from build123d import *

# Parameters (mm, degrees)
F0_R     = 203.2
F0_R_2   = 8.89
F1_DEPTH = 20.32


with BuildPart() as f1:
    # F0 (on Front) → F1 (new body)
    with BuildSketch(Plane.XZ):
        Circle(F0_R)
        with Locations((-134.703841816, -134.703841816)):
            Circle(F0_R_2, mode=Mode.SUBTRACT)
        with Locations((0, -190.5)):
            Circle(F0_R_2, mode=Mode.SUBTRACT)
        with Locations((-190.5, 0)):
            Circle(F0_R_2, mode=Mode.SUBTRACT)
        with Locations((134.703841816, -134.703841816)):
            Circle(F0_R_2, mode=Mode.SUBTRACT)
        with Locations((190.5, 0)):
            Circle(F0_R_2, mode=Mode.SUBTRACT)
        with BuildLine():
            ThreePointArc((-123.8970573285, 144.2619540188), (-120.3869637363, 158.4652267944), (-108.347947169, 150.1516358339))
            ThreePointArc((-108.347947169, 150.1516358339), (-114.0889306017, 141.8380448734), (-123.8970573285, 144.2619540188))
        make_face(mode=Mode.SUBTRACT)
        with Locations((0, 190.5)):
            Circle(F0_R_2, mode=Mode.SUBTRACT)
        with Locations((117.237947169, 150.1516358339)):
            Circle(F0_R_2, mode=Mode.SUBTRACT)
    extrude(amount=F1_DEPTH)


solid = f1.part
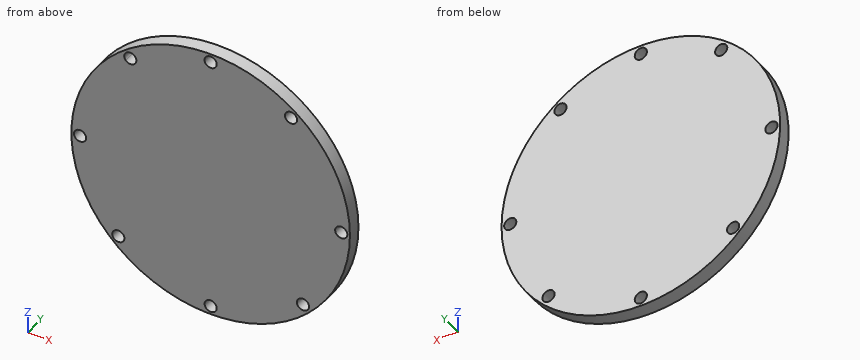
Could you check a few things on this model? Use its own coordinates, in mm. Coordinates: 2 decimals unless noted, no trailing zeros. Order: outer loops, then holes, each group sorted by start corner. A loop starts at its lowest first (then second) coordinate and runs counter-clockwise, first axis right, second up. Notation, with made-up numbers: (66.25, 32.25) - (105.25, 32.25) arc R12 cw to (105.25, 42.25) - close; hole circle Ø4 at (62, -12). An arc over 180 degrees is marked (long way). Answer in a Markdown table with one row per item. Add a question column.
(1) If we section it at A-A, the plane z = 0: Please give me the cut outline in (x, y), then the cut area to 3 significant figures.
(2) If we section it at D-D, the plane z = -190.5: Please give me the cut outline in (x, y), then the cut area to 3 significant figures.
(3) Will these pins go through, and if not, where does the flat tip stop? pin 1 (10.5 mm diameter, centred on x = -190.5, z = 0, fed in from +Y); pin 2 (1.5 mm diameter, centred on y = -15.5, z = -116, fed in from +X); pin 3 (5 mm diameter, centred on y = -16.5, z = 12.5, fed in from -X); pin 4 (1.5 mm diameter, centred on y = -10.5, z = 25, fed in from +X).
(4) If we section it at C-C, the plane y = -10.5: State how many separate pieces and enclosed holes the cut face has, then the cut area to 3 significant figures.
(5) If we section it at B-B, the plane x = 119: Please give me the cut outline in (y, z), then the cut area to 3 significant figures.
(6) I need wall thicknesses on L1, parallel to Z at x = 0, y = -15.75; L2, parallel to X at y = -8.5, z = 148; L3, parallel to Z at x = -127, y = -11.5. Which ranges of each line are inside material? Lowest first, please.
Results are:
| question | item | result |
|---|---|---|
| 1 | outline | (-203.2, -20.32) - (-199.39, -20.32) - (-199.39, 0) - (-203.2, 0) - close; (-181.61, -20.32) - (181.61, -20.32) - (181.61, 0) - (-181.61, 0) - close; (199.39, -20.32) - (203.2, -20.32) - (203.2, 0) - (199.39, 0) - close |
| 1 | area | 7,540 mm2 |
| 2 | outline | (-70.71, -20.32) - (-8.89, -20.32) - (-8.89, 0) - (-70.71, 0) - close; (8.89, -20.32) - (70.71, -20.32) - (70.71, 0) - (8.89, 0) - close |
| 2 | area | 2,510 mm2 |
| 3 | pin 1 | passes through |
| 3 | pin 2 | stops at x = 167.35 |
| 3 | pin 3 | stops at x = -202.95 |
| 3 | pin 4 | stops at x = 201.75 |
| 4 | separate pieces | 1 |
| 4 | enclosed holes | 8 |
| 4 | area | 128,000 mm2 |
| 5 | outline | (-20.32, -164.71) - (0, -164.71) - (0, 141.44) - (-20.32, 141.44) - close; (-20.32, 158.87) - (0, 158.87) - (0, 164.71) - (-20.32, 164.71) - close |
| 5 | area | 6,340 mm2 |
| 6 | L1 | z = -203.2 to -199.39, -181.61 to 181.61, 199.39 to 203.2 |
| 6 | L2 | x = -139.23 to -125.86, -108.61 to 108.61, 125.86 to 139.23 |
| 6 | L3 | z = -158.62 to -139.14, -130.27 to 158.62 |
